Could you check a few things on this model? Use its own coordinates, in mm. A direction names the side the tool comes from. Give positions to 0.01 mm unless a question says otherwise; leave off trailing zeros. Order: outer loops, then holes, each group sorted by start corner. A loop starts at its lowest first (then second) coordinate and runs counter-clockwise, first axis right, second up.
from build123d import *

# Parameters (mm, degrees)
SKETCH1_R           = 53.721
BOSS_EXTRUDE1_DEPTH = 4.7625
CUT_EXTRUDE1_REACH  = 78.122
CUT_EXTRUDE2_REACH  = 77.801


with BuildPart() as part:
    # Sketch1 → Boss-Extrude1 (new body)
    with BuildSketch(Plane(origin=(0, 0, 0), x_dir=(1, 0, 0), z_dir=(0, 1, 0))):
        with Locations(Location((0, 0, 0), (0, 0, 90))):
            Circle(SKETCH1_R)
    extrude(amount=BOSS_EXTRUDE1_DEPTH)

    # Sketch2 → Cut-Extrude1 (cut, up to next)
    with BuildSketch(Plane(origin=(0, 4.7625, 0), x_dir=(1, 0, 0), z_dir=(0, 1, 0)), mode=Mode.PRIVATE) as cut_extrude1_sk1:
        with BuildLine():
            Line((-6.985, -48.184956735), (6.985, -48.184956735))
            Line((6.985, -48.184956735), (6.985, -53.264956735))
            ThreePointArc((6.985, -53.264956735), (0, -53.721), (-6.985, -53.264956735))
            Line((-6.985, -53.264956735), (-6.985, -48.184956735))
        make_face()
    cut_extrude1_tool1 = extrude(cut_extrude1_sk1.sketch, amount=-CUT_EXTRUDE1_REACH, mode=Mode.PRIVATE) & part.part
    # Sketch2 → Cut-Extrude1 (cut, up to next)
    with BuildSketch(Plane(origin=(0, 4.7625, 0), x_dir=(1, 0, 0), z_dir=(0, 1, 0)), mode=Mode.PRIVATE) as cut_extrude1_sk2:
        with BuildLine():
            Line((6.985, 48.184956735), (6.985, 53.264956735))
            ThreePointArc((6.985, 53.264956735), (0, 53.721), (-6.985, 53.264956735))
            Line((-6.985, 53.264956735), (-6.985, 48.184956735))
            Line((-6.985, 48.184956735), (6.985, 48.184956735))
        make_face()
    cut_extrude1_tool2 = extrude(cut_extrude1_sk2.sketch, amount=-CUT_EXTRUDE1_REACH, mode=Mode.PRIVATE) & part.part
    add(cut_extrude1_tool1.solids().sort_by_distance((0, 4.7625, 50.878815))[0], mode=Mode.SUBTRACT)
    add(cut_extrude1_tool2.solids().sort_by_distance((0, 4.7625, -50.878815))[0], mode=Mode.SUBTRACT)

    # Sketch3 → Cut-Extrude2 (cut, up to next)
    with BuildSketch(Plane(origin=(0, 4.7625, 0), x_dir=(1, 0, 0), z_dir=(0, 1, 0)), mode=Mode.PRIVATE) as cut_extrude2_sk1:
        with BuildLine():
            Line((38.236896613, -30.141665813), (45.221896613, -18.043290922))
            Line((45.221896613, -18.043290922), (49.621305664, -20.583290922))
            ThreePointArc((49.621305664, -20.583290922), (46.523750717, -26.8605), (42.636305664, -32.681665813))
            Line((42.636305664, -32.681665813), (38.236896613, -30.141665813))
        make_face()
    cut_extrude2_tool1 = extrude(cut_extrude2_sk1.sketch, amount=-CUT_EXTRUDE2_REACH, mode=Mode.PRIVATE) & part.part
    # Sketch3 → Cut-Extrude2 (cut, up to next)
    with BuildSketch(Plane(origin=(0, 4.7625, 0), x_dir=(1, 0, 0), z_dir=(0, 1, 0)), mode=Mode.PRIVATE) as cut_extrude2_sk2:
        with BuildLine():
            Line((-45.221896613, 18.043290922), (-49.621305664, 20.583290922))
            ThreePointArc((-49.621305664, 20.583290922), (-46.523750717, 26.8605), (-42.636305664, 32.681665813))
            Line((-42.636305664, 32.681665813), (-38.236896613, 30.141665813))
            Line((-38.236896613, 30.141665813), (-45.221896613, 18.043290922))
        make_face()
    cut_extrude2_tool2 = extrude(cut_extrude2_sk2.sketch, amount=-CUT_EXTRUDE2_REACH, mode=Mode.PRIVATE) & part.part
    add(cut_extrude2_tool1.solids().sort_by_distance((44.062347, 4.7625, 25.439408))[0], mode=Mode.SUBTRACT)
    add(cut_extrude2_tool2.solids().sort_by_distance((-44.062347, 4.7625, -25.439408))[0], mode=Mode.SUBTRACT)


solid = part.part
Item 1: Imagine slicing it at A-A on y = 3.75. List the corners of the cut face in (x, z) for me (3 decimals).
Findings:
outline: (-49.621, -20.583) - (-45.222, -18.043) - (-38.237, -30.142) - (-42.636, -32.682) arc R53.721 ccw to (-6.985, -53.265) - (-6.985, -48.185) - (6.985, -48.185) - (6.985, -53.265) arc R53.721 ccw to (49.621, 20.583) - (45.222, 18.043) - (38.237, 30.142) - (42.636, 32.682) arc R53.721 ccw to (6.985, 53.265) - (6.985, 48.185) - (-6.985, 48.185) - (-6.985, 53.265) arc R53.721 ccw to start
Item 2: Imagine slicing it at B-B on x = -5.5. List the corners of the cut face in (y, z) for me.
Findings:
outline: (0, -48.18) - (4.76, -48.18) - (4.76, 48.18) - (0, 48.18) - close
Item 3: For pin 1 (1.4 mm diameter, centred on y = 3.5, z = -49.5, fed in from +X); pin 2 (1.5 mm diameter, centred on y = 4, z = 35.5, fed in from -X); pin 3 (1.4 mm diameter, centred on x = 2, y = 2.5, fed in from +Z), each with a flat end and sliding along its axis, tell me the tip position at first contact or that it passes through.
Findings:
pin 1: stops at x = 22.46
pin 2: stops at x = -40.97
pin 3: stops at z = 48.18
Item 4: Please list where these lines run through material, in increasing order: line 1 along Z through (x, y) = (-3, 0.8); line 2 along Z through (x, y) = (40, 0.75); line 3 along Z through (x, y) = (42.5, 4.4).
Findings:
line 1: z = -48.18 to 48.18
line 2: z = -35.86 to 27.09, 31.16 to 35.86
line 3: z = -32.86 to 22.76, 32.6 to 32.86
Item 5: For faces 4 (the flat face through (-40.47, 2.41, -31.43)), 5 (the flat face through (41.68, 2.41, 24.18)), 6 (the cylindrical face through (-26.604, 2.348, -46.671)), 7 (the flat face through (-6.985, 2, 51)), 8 (the flat face through (6.985, 2, -51)), which set-ups out of +Z, -Z, +X, -X, +Y, -Y let a thin tool reach every point of the face, with its end or its side?
Findings:
face 4: -X, +Y, -Y
face 5: +Y, -Y
face 6: -Z, -X, +Y, -Y
face 7: +Z, +Y, -Y
face 8: -Z, +Y, -Y
Item 6: Imagine slicing it at C-C on z = 45. List the corners of the cut face in (x, y) for me, then the cut area to 3 significant figures.
Findings:
outline: (-29.34, 0) - (29.34, 0) - (29.34, 4.76) - (-29.34, 4.76) - close
area: 279 mm2
Item 7: We'd pull the mould along Z, two halves only. Please class faces 1 (the flat face through (47.4, 2.4, 19.3)), 2 (the flat face through (-1, 0, 1)), 3 (the flat face through (40.47, 2.41, 31.43)): +Z half, -Z half, draft (parallel to the pull), parting line (faces both ways), or undercut.
Findings:
face 1: +Z half
face 2: draft
face 3: undercut
